Can you work these out from the model? Positions are in its coordinate system, mm. Round coordinates to 2 decimals unless told otherwise and drop trailing zeros. Order: outer loops, then holes, each group sorted by start corner. A loop starts at its lowest first (then second) coordinate and runs counter-clockwise, first axis right, second up.
Q1. If we section it at A-A (y = 4): Please give me the cut outline in (x, z).
Q2. Will these pins go through, and if not, where does the flat tip stop? P1, Ø2, axis at x = 10, y = -10.5, coming from the +Z side; P2, Ø2, axis at x = 10.7, y = 10.7, coming from the -Z side.
Q3. If we section it at C-C (x = -10.7): Please give me the cut outline in (y, z).
Q4. If I drill on line 1 (Y direction, x = -10.7, z = 1.2); line 2 (Y direction, x = -3, z = 2.9); line 3 (X direction, y = -10, z = 2.9), over which ranges is the centre line in solid material (lowest first)?
Q5. If we section it at B-B (z = 3.8): Count the separate pieces of the cut face and the enclosed holes in it, plus the area to 3 significant figures.
from build123d import *

# Parameters (mm, degrees)
BOSS_EXTRUDE1_DEPTH            = 5
F_1_0MM_DOWEL_HOLE1_D          = 1
CBORE_FOR_M2_SHCS1_D           = 2.6
CBORE_FOR_M2_SHCS1_CBORE_D     = 4.4
CBORE_FOR_M2_SHCS1_CBORE_DEPTH = 2


with BuildPart() as part:
    # Sketch1 → Boss-Extrude1 (new body)
    with BuildSketch(Plane.XY):
        with BuildLine():
            Line((-12.7, 12.7), (-12.7, -11.7))
            ThreePointArc((-12.7, -11.7), (-12.407106781, -12.407106781), (-11.7, -12.7))
            Line((-11.7, -12.7), (11.7, -12.7))
            ThreePointArc((11.7, -12.7), (12.407106781, -12.407106781), (12.7, -11.7))
            Line((12.7, -11.7), (12.7, 12.7))
            Line((12.7, 12.7), (-12.7, 12.7))
        make_face()
    extrude(amount=BOSS_EXTRUDE1_DEPTH)

    # Ø1.0mm Dowel Hole1 (through all)
    with Locations(Plane.XY.offset(5)):
        with Locations((3, -4), (-3, -4), (-3, 4), (3, 4)):
            Hole(F_1_0MM_DOWEL_HOLE1_D / 2)

    # CBORE for M2 SHCS1 (through all)
    with Locations(Plane.XY.offset(5)):
        with Locations((10.7, -10.7), (-10.7, -10.7), (-10.7, 10.7), (10.7, 10.7)):
            CounterBoreHole(CBORE_FOR_M2_SHCS1_D / 2, CBORE_FOR_M2_SHCS1_CBORE_D / 2, CBORE_FOR_M2_SHCS1_CBORE_DEPTH)


solid = part.part
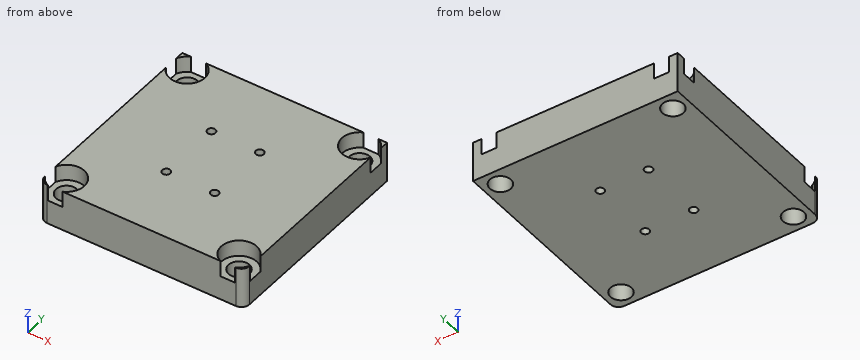
Solution:
1. outline: (-12.7, 0) - (-3.5, 0) - (-3.5, 5) - (-12.7, 5) - close; (-2.5, 0) - (2.5, 0) - (2.5, 5) - (-2.5, 5) - close; (3.5, 0) - (12.7, 0) - (12.7, 5) - (3.5, 5) - close
2. P1: stops at z = 3
2. P2: passes through
3. outline: (-12.7, 0) - (-12, 0) - (-12, 3) - (-12.7, 3) - close; (-9.4, 0) - (9.4, 0) - (9.4, 3) - (8.5, 3) - (8.5, 5) - (-8.5, 5) - (-8.5, 3) - (-9.4, 3) - close; (12, 0) - (12.7, 0) - (12.7, 3) - (12, 3) - close
4. line 1: y = -12.7 to -12, -9.4 to 9.4, 12 to 12.7
4. line 2: y = -12.7 to -4.5, -3.5 to 3.5, 4.5 to 12.7
4. line 3: x = -12.7 to -11.8, -9.6 to 9.6, 11.8 to 12.7
5. separate pieces: 5
5. enclosed holes: 4
5. area: 583 mm2
